For this review, use the dimensioned drawing (mm, ordinates from the lowest corner) and the shaded views. Coordinates: 2 decimals unless noted, no trailing zeros. Loops run counter-clockwise (first coordinate to the right, second up) from the corner with the lowest first, then second, coordinate; pieces in that order, holes last. Notation, with made-up numbers: (54.5, 43) -> (64.5, 43) arc R19 ccw to (64.5, 71) -> close; hole circle Ø8 at (71.5, 5.25). An arc over 180 degrees is marked (long way). Use one line per item in the form item = value. Start each with the question number.
1. Consider section C-C (y = 13.5). State the section outline as (x, z) points, then the cut area to 3 significant figures.
2. Wall thickness on line 1 (Z direction, x = 53, y = 1.5); line 2 (Y direction, x = 53, z = 14); line 3 (X direction, y = 4, z = 7): over which ranges is each line inside the solid? List them lowest first. Write a range as from..to.
3. Consider section D-D (z = 16). State the section outline as (x, y) points.
4. Consider section B-B (z = 6). State the section outline as (x, y) points.
5. Consider section A-A (x = 30). State the section outline as (y, z) points.
6. The part is to be moulded in two halves that separate along X. For the marked faces 1, 2 and 3, say which applies: released by +X, released by -X, zero draft, split by the parting line, or undercut.
7. For pin 1 (3.5 mm diameter, centred on x = 53, z = 25, fed in from -Y), flat-tipped, find the tip position at first contact; note if it passes through.
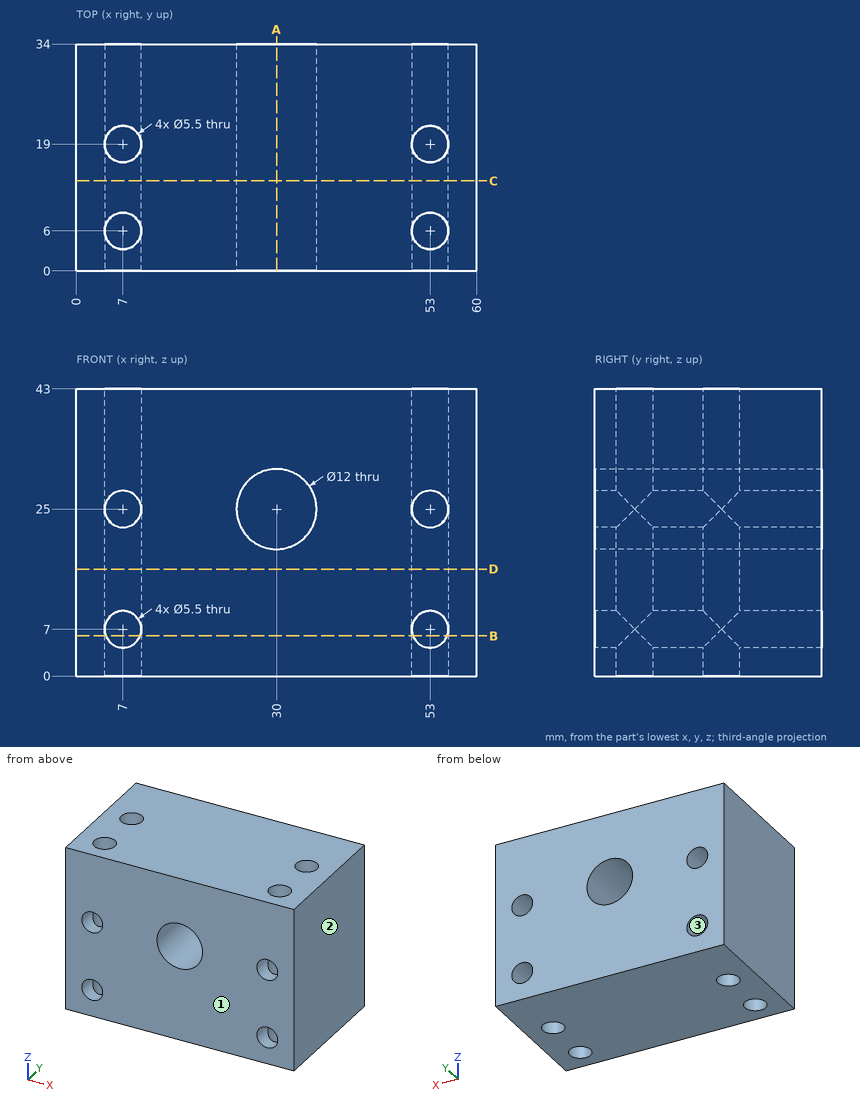
Geometry check:
q1.outline = (0, 0) -> (60, 0) -> (60, 43) -> (0, 43) -> close; hole circle Ø5.5 at (7, 7); hole circle Ø5.5 at (7, 25); hole circle Ø12 at (30, 25); hole circle Ø5.5 at (53, 7); hole circle Ø5.5 at (53, 25)
q1.area = 2,370 mm²
q2.line_1 = 0..4.25, 9.75..22.25, 27.75..43
q2.line_2 = 0..3.25, 8.75..16.25, 21.75..34
q2.line_3 = 0..4.25, 9.75..50.25, 55.75..60
q3.outline = (0, 0) -> (60, 0) -> (60, 34) -> (0, 34) -> close; hole circle Ø5.5 at (7, 6); hole circle Ø5.5 at (7, 19); hole circle Ø5.5 at (53, 6); hole circle Ø5.5 at (53, 19)
q4.outline = (0, 0) -> (4.44, 0) -> (4.44, 5) arc R2.75 cw to (4.44, 7) -> (4.44, 18) arc R2.75 cw to (4.44, 20) -> (4.44, 34) -> (0, 34) -> close; (9.56, 0) -> (50.44, 0) -> (50.44, 5) arc R2.75 cw to (50.44, 7) -> (50.44, 18) arc R2.75 cw to (50.44, 20) -> (50.44, 34) -> (9.56, 34) -> (9.56, 20) arc R2.75 cw to (9.56, 18) -> (9.56, 7) arc R2.75 cw to (9.56, 5) -> close; (55.56, 0) -> (60, 0) -> (60, 34) -> (55.56, 34) -> (55.56, 20) arc R2.75 cw to (55.56, 18) -> (55.56, 7) arc R2.75 cw to (55.56, 5) -> close
q5.outline = (0, 0) -> (34, 0) -> (34, 19) -> (0, 19) -> close; (0, 31) -> (34, 31) -> (34, 43) -> (0, 43) -> close
q6.face_1 = zero draft
q6.face_2 = released by +X
q6.face_3 = undercut
q7.pin_1 = through
